Source: three-view drawing plus pictorial views. Frame: mm from the lowest corner of the part. A direction names the side the tool comes from. Give positions to 0.01 mm unless a question says otherwise; leave off trailing zeros. Write each loop counter-clockwise with the first axis right and the second up, starting at its lowest first coordinate (ties: lowest second). Pieces come first, ordered by that corner, then holes.
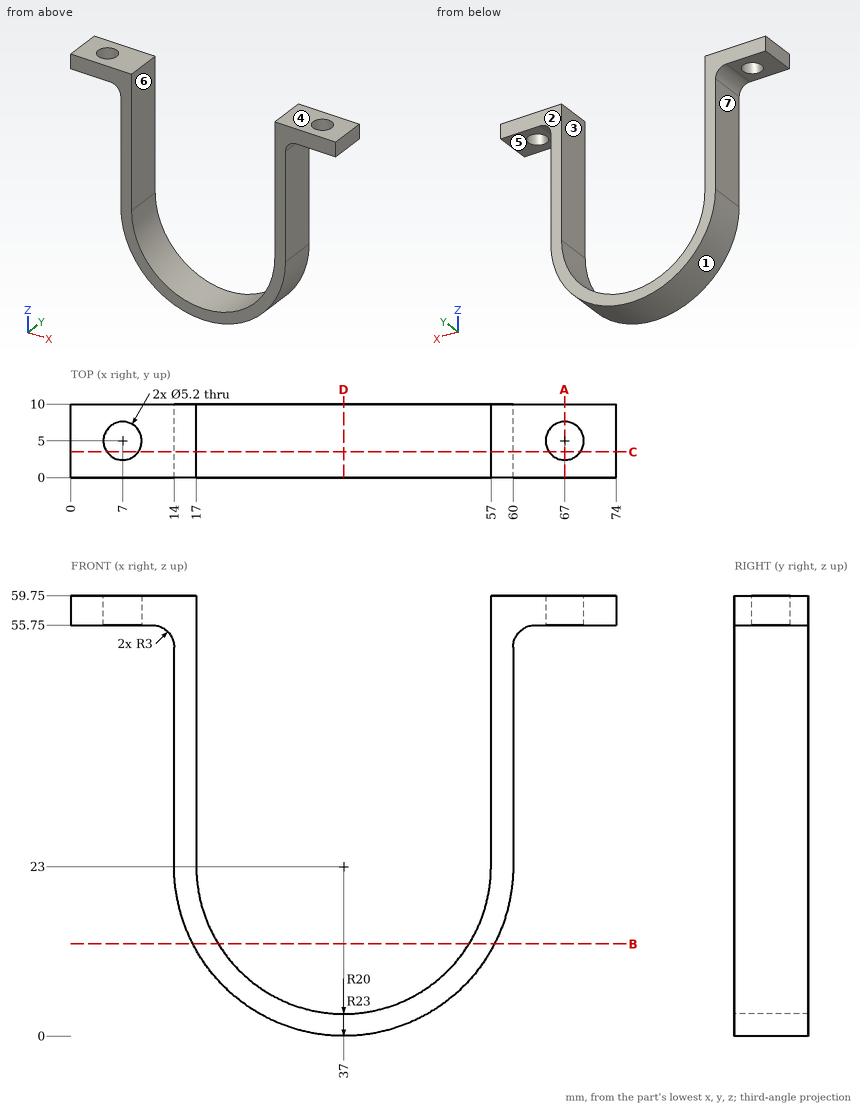
Q1. Access query for the marked faces 4, 5, 6 and 7. Directions: +Z, -Z, +X, -X, +Y, -Y. A direction counts if a zero-diameter tool reaches every point of the face in a straight line with its end or side. Return the directions, or none.
Filled sheet:
face 4: +Z, +X, -X, +Y, -Y
face 5: -Z, +X, +Y, -Y
face 6: +Z, +Y, -Y
face 7: -Z, -X, +Y, -Y
Q2. Section A-A on x = 67. Output: boundary loops of the cut face in (y, z).
Filled sheet:
outline: (0, 55.75) - (2.4, 55.75) - (2.4, 59.75) - (0, 59.75) - close; (7.6, 55.75) - (10, 55.75) - (10, 59.75) - (7.6, 59.75) - close
Q3. Ray query, line 1 along Y through (x, z) = (67, 57.1); line 2 along X through (y, z) = (3, 31); line 3 along Z through (x, y) = (69.5, 2). Return the intervals inside material, ascending.
Filled sheet:
line 1: y = 0 to 2.4, 7.6 to 10
line 2: x = 14 to 17, 57 to 60
line 3: z = 55.75 to 59.75
Q4. Section D-D on x = 37. Output: boundary loops of the cut face in (y, z), plus the area to 3 significant figures.
Filled sheet:
outline: (0, 0) - (10, 0) - (10, 3) - (0, 3) - close
area: 30.0 mm2
Q5. Pin query (flat end, axial travel): P1, Ø4, axis at x = 45.5, y = 3.5, coming from the -Z side; P2, Ø1.5, axis at y = 5.5, z = 34, coming from the +X side; P3, Ø5, axis at x = 69.5, y = 7, coming from the -Z side. Return the tip coordinate at first contact, or that it passes through.
Filled sheet:
P1: stops at z = 0.94
P2: stops at x = 60
P3: stops at z = 55.75
Q6. Section B-B on z = 12.5. Output: boundary loops of the cut face in (x, y), plus the area to 3 significant figures.
Filled sheet:
outline: (16.54, 0) - (19.98, 0) - (19.98, 10) - (16.54, 10) - close; (54.02, 0) - (57.46, 0) - (57.46, 10) - (54.02, 10) - close
area: 68.8 mm2
Q7. Section C-C on y = 3.5. Output: boundary loops of the cut face in (x, z).
Filled sheet:
outline: (0, 55.75) - (4.88, 55.75) - (4.88, 59.75) - (0, 59.75) - close; (9.12, 55.75) - (11, 55.75) arc R3 cw to (14, 52.75) - (14, 23) arc R23 ccw to (60, 23) - (60, 52.75) arc R3 cw to (63, 55.75) - (64.88, 55.75) - (64.88, 59.75) - (57, 59.75) - (57, 23) arc R20 cw to (17, 23) - (17, 59.75) - (9.12, 59.75) - close; (69.12, 55.75) - (74, 55.75) - (74, 59.75) - (69.12, 59.75) - close
Q8. Pull-direction query (X, two-part tool) for the marked faces 1, 2 and 3; classes: released by +X, released by -X, zero draft, split by the parting line, or undercut.
Filled sheet:
face 1: split by the parting line
face 2: zero draft
face 3: undercut
